```python
from build123d import *

# Parameters (mm, degrees)
SKETCH1_R  = 0.95
BODY_DEPTH = 8.1
LOCK_DEPTH = 1


with BuildPart() as part:
    # Sketch1 → Body (new body)
    with BuildSketch(Plane(origin=(0, 0, 0), x_dir=(1, 0, 0), z_dir=(0, 1, 0))):
        Circle(SKETCH1_R)
    extrude(amount=BODY_DEPTH)

    # Sketch2 → Lock (add)
    with BuildSketch(Plane(origin=(0, 8.1, 0), x_dir=(1, 0, 0), z_dir=(0, 1, 0))):
        with BuildLine():
            ThreePointArc((-0.807774721, -0.5), (-0.95, 0), (-0.807774721, 0.5))
            Line((-0.807774721, 0.5), (-1.9, 0.5))
            Line((-1.9, 0.5), (-1.9, -0.5))
            Line((-1.9, -0.5), (-0.807774721, -0.5))
        make_face()
        with BuildLine():
            Line((1.9, 0.5), (0.807774721, 0.5))
            ThreePointArc((0.807774721, 0.5), (0.91375215, 0.259917309), (0.95, 0))
            ThreePointArc((0.95, 0), (0.91375215, -0.259917309), (0.807774721, -0.5))
            Line((0.807774721, -0.5), (1.9, -0.5))
            Line((1.9, -0.5), (1.9, 0.5))
        make_face()
    extrude(amount=-LOCK_DEPTH)


solid = part.part
```
Check sheet for the modelled part. Datum: model origin and axes. Units: mm. A direction names the side the tool comes from. Coordinates: 2 decimals unless noted, no trailing zeros. Order: outer loops, then holes, each group sorted by start corner. A loop starts at its lowest first (then second) coordinate and runs counter-clockwise, first axis right, second up. Notation, with made-up numbers: (4, -22.5) -> (34, -22.5) arc R16 cw to (34, -11.5) -> close; hole circle Ø11 at (7.5, 85). An arc over 180 degrees is marked (long way). Write item = value, one per line. Start each with the question number.
1) Cross-section at C-C (x = -1.1). Enter the section's corners in (y, z), then the cut area to 3 significant figures.
2) Go/stop test with flat-tipped pins: P1, Ø1.1, axis at x = 1, y = 7.5, coming from the +Z side; P2, Ø0.5, axis at x = 1, y = 7.5, coming from the -Z side; P3, Ø0.8, axis at x = -1.5, y = 8, coming from the -Z side. Record where each tip stops, or that it passes through.
3) Material ranges on L1, parallel to Y at x = -1.5, z = -0.15; L2, parallel to X at y = 1, z = -0.5; L3, parallel to X at y = 3.5, z = 0.2, recorded low to high.
4) Cross-section at D-D (z = -0.4). Enter the section's corners in (x, y), then the cut area to 3 significant figures.
5) Cross-section at A-A (z = 0). Enter the section's corners in (x, y).
6) Cross-section at B-B (y = 5.25). Enter the section's corners in (x, z).
7) Access from +Z, -Z, +X, -X, +Y, -Y to the whole of each face (thin tool, end or side, straight path). Record for faces 1 (the flat face through (-1.4, 7.6, 0.5)), 2 (the flat face through (-1.3, 7.6, -0.5)), 3 (the cylindrical face through (-0.95, 3.99, -0.04)), 4 (the flat face through (1.3, 7.6, 0.5)).
Ans:
q1.outline = (7.1, -0.5) -> (8.1, -0.5) -> (8.1, 0.5) -> (7.1, 0.5) -> close
q1.area = 1.00 mm²
q2.P1 = 0.84
q2.P2 = -0.58
q2.P3 = -0.5
q3.L1 = 7.1 to 8.1
q3.L2 = -0.81 to 0.81
q3.L3 = -0.93 to 0.93
q4.outline = (-1.9, 7.1) -> (-0.86, 7.1) -> (-0.86, 0) -> (0.86, 0) -> (0.86, 7.1) -> (1.9, 7.1) -> (1.9, 8.1) -> (-1.9, 8.1) -> close
q4.area = 16.0 mm²
q5.outline = (-1.9, 7.1) -> (-0.95, 7.1) -> (-0.95, 0) -> (0.95, 0) -> (0.95, 7.1) -> (1.9, 7.1) -> (1.9, 8.1) -> (-1.9, 8.1) -> close
q6.outline = circle Ø1.9 at (0, 0)
q7.face_1 = +Z, -X, +Y, -Y
q7.face_2 = -Z, -X, +Y, -Y
q7.face_3 = -Y
q7.face_4 = +Z, +X, +Y, -Y
